Autodesk Inventor part; units mm, degrees
ref_plane "YZ Plane" through (0, 0, 0) normal (1, 0, 0) x (0, 1, 0)
ref_plane "XZ Plane" through (0, 0, 0) normal (0, 1, 0) x (-1, 0, 0)
ref_plane "XY Plane" through (0, 0, 0) normal (0, 0, 1) x (1, 0, 0)
sketch "Boceto1" plane through (0, 0, 0) normal (0, 0, 1) x (1, 0, 0)
  line L0 (0, 0) -> (127.5, 0)
  line L1 (127.5, 0) -> (127.5, 177)
  line L2 (127.5, 177) -> (0, 177)
  line L3 (0, 177) -> (0, 0)
  dimension "d32" = 127.5
  dimension "d33" = 177
extrude "Extrusión1" add sketch "Boceto1" along normal blind 2.5
sketch "Boceto2" plane through (0, 0, 2.5) normal (0, 0, 1) x (1, 0, 0)
  line L0 (127.5, 0) -> (127.5, 27.5)
  line L1 (127.5, 0) -> (127.5, 177)
  line L2 (127.5, 0) -> (155, 0) construction
  line L3 (127.5, 27.5) -> (113.75, 27.5)
  line L4 (0, 0) -> (127.5, 0)
  line L5 (113.75, 27.5) -> (13.75, 27.5)
  line L6 (13.75, 27.5) -> (13.75, 149.5)
  line L7 (13.75, 149.5) -> (113.75, 149.5)
  line L8 (113.75, 149.5) -> (113.75, 27.5)
  dimension "d36" = 27.5
  dimension "d37" = 90
  dimension "d38" = 13.75
  dimension "d39" = 90
  dimension "d40" = 100
  dimension "d41" = 122
extrude "Extrusión2" cut sketch "Boceto2" against normal blind 2.5
sketch "Boceto3" plane through (0, 0, 2.5) normal (0, 0, 1) x (1, 0, 0)
  line L0 (13.75, 149.5) -> (7.75, 149.5)
  line L1 (7.75, 149.5) -> (7.75, 155.5)
  line L2 (113.75, 27.5) -> (113.75, 21.5)
  line L3 (113.75, 27.5) -> (119.75, 27.5) construction
  line L4 (113.75, 21.5) -> (119.75, 21.5)
  line L5 (7.75, 155.5) -> (119.75, 155.5)
  line L6 (119.75, 155.5) -> (119.75, 21.5)
  line L7 (119.75, 21.5) -> (7.75, 21.5)
  line L8 (7.75, 21.5) -> (7.75, 155.5)
  line L9 (0, 177) -> (127.5, 177)
  line L10 (127.5, 177) -> (127.5, 0)
  line L11 (127.5, 0) -> (0, 0)
  line L12 (0, 0) -> (0, 177)
  dimension "d44" = 6
  dimension "d45" = 6
  dimension "d46" = 90
  dimension "d47" = 6
  dimension "d48" = 90
  dimension "d49" = 6
  dimension "d50" = 90
extrude "Extrusión3" add sketch "Boceto3" along normal blind 6
sketch "Boceto6" plane through (0, 0, 8.5) normal (0, 0, 1) x (1, 0, 0)
  line L0 (0, 0) -> (0, 88.5)
  line L1 (0, 177) -> (0, 0)
  line L2 (0, 0) -> (88.5, 0) construction
  line L3 (0, 88.5) -> (127.5, 88.5)
  dimension "d73" = 88.5
  dimension "d74" = 90
  dimension "d75" = 127.5
  dimension "d76" = 90
ref_plane "Plano de trabajo1" through (0, 88.5, 8.5) normal (0, -1, 0) x (1, 0, 0)
sketch "Boceto7" plane through (0, 0, 8.5) normal (0, 0, 1) x (1, 0, 0)
  line L0 (0, 0) -> (63.75, 0)
  line L1 (0, 0) -> (127.5, 0)
  line L2 (63.75, 0) -> (63.75, 177)
  line L3 (127.5, 177) -> (0, 177)
  line L4 (63.75, 0) -> (240.75, 0) construction
  dimension "d78" = 177
  dimension "d79" = 90
ref_plane "Plano de trabajo2" through (63.75, 0, 8.5) normal (1, 0, 0) x (0, 1, 0)
sketch "Boceto8" plane through (0, 0, 2.5) normal (0, 0, 1) x (1, 0, 0)
  line L0 (13.75, 27.5) -> (7.75, 27.5)
  line L1 (7.75, 27.5) -> (7.75, 21.5)
  line L2 (7.75, 21.5) -> (13.75, 21.5)
  line L3 (13.75, 21.5) -> (13.75, 27.5)
  line L4 (13.75, 21.5) -> (7.75, 27.5)
  line L5 (13.75, 27.5) -> (7.75, 21.5)
  circle A0 centre (10.75, 24.5) radius 1.6
  point P0 (0, 0)
  dimension "d81" = 6
  dimension "d82" = 6
  dimension "d83" = 3.2
extrude "Extrusión4" cut sketch "Boceto8" against normal blind 4 contours A0 L4 L5 | L5 L4 A0 | L4 L5 A0 | A0 L5 L4
mirror "Simetría1" about plane through (63.75, 0, 8.5) normal (1, 0, 0) of "Extrusión4"
mirror "Simetría2" about plane through (0, 88.5, 8.5) normal (0, -1, 0) of "Extrusión4", "Simetría1"
sketch "Boceto9" plane through (0, 0, 8.5) normal (0, 0, 1) x (1, 0, 0)
  line L0 (0, 177) -> (11.5, 177)
  line L1 (11.5, 177) -> (11.5, 165.5)
  line L2 (11.5, 165.5) -> (0, 165.5)
  line L3 (0, 165.5) -> (0, 177)
  line L4 (0, 177) -> (11.5, 165.5)
  line L5 (0, 165.5) -> (11.5, 177)
  circle A0 centre (5.75, 171.25) radius 2.1
  point P0 (0, 0)
  dimension "d86" = 11.5
  dimension "d87" = 11.5
  dimension "d88" = 4.2
extrude "Extrusión5" cut sketch "Boceto9" against normal blind 10 contours A0 L5 L4 | L4 L5 A0 | A0 L4 L5 | L5 L4 A0
mirror "Simetría3" about plane through (63.75, 0, 8.5) normal (1, 0, 0) of "Extrusión5"
mirror "Simetría4" about plane through (0, 88.5, 8.5) normal (0, -1, 0) of "Extrusión5", "Simetría3"
properties part number "transillum_diffusor_partA_v3"
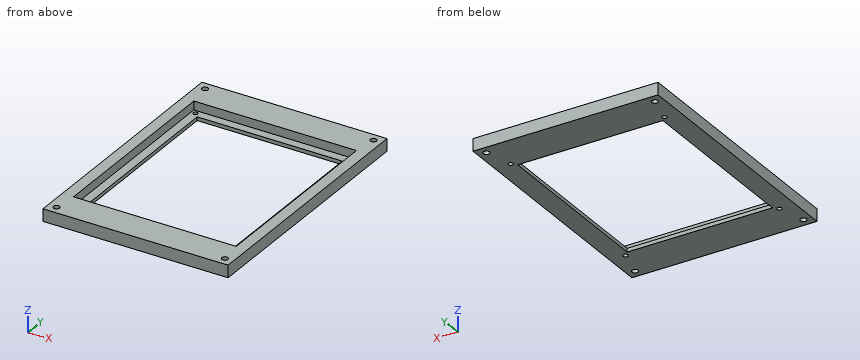
Can you work these out from the model? Positions are in its coordinate system, mm. Round coordinates to 2 decimals unless told otherwise and drop trailing zeros. Write each loop counter-clockwise with the first axis right and the second up, starting at its lowest first coordinate (ties: lowest second). Pieces come first, ordered by that corner, then holes. Notation, with made-up numbers: (35.5, -7) -> (71.5, -7) arc R24 ccw to (71.5, 23) -> close; hole circle Ø9 at (31, 21). An arc over 180 degrees is marked (long way). One line per question, with ' | ' between items. Start each with the question number.
1) Suppose I cut it at A-A on x = 107. Write out the boundary of the cut face in (y, z), then the cut area to 4 significant figures.
2) I need wall thicknesses on line 1 (Y direction, x = 5.75, z = 4); line 2 (X direction, y = 171.25, z = 5.5); line 3 (Y direction, x = 10.75, z = 1.75). Which ranges of each line are inside material? Lowest first, please. Write a range as [from, to].
3) I'm going to push flat-ended pins straight in: P1, Ø4, axis at x = 10.75, y = 152.5, coming from the -Z side; P2, Ø1, axis at x = 16, y = 153.5, coming from the +Z side. Where does each tip first touch, or does it pass through?
4) Suppose I cut it at C-C on y = 89. Write out the boundary of the cut face in (x, z), then the cut area to 3 significant figures.
5) Suppose I cut it at B-B on y = 5.75. Write out the boundary of the cut face in (x, z), then the cut area to 3 significant figures.
Return value:
1) outline: (0, 0) -> (27.5, 0) -> (27.5, 2.5) -> (21.5, 2.5) -> (21.5, 8.5) -> (0, 8.5) -> close; (149.5, 0) -> (177, 0) -> (177, 8.5) -> (155.5, 8.5) -> (155.5, 2.5) -> (149.5, 2.5) -> close | area: 395.5 mm2
2) line 1: y = [0, 3.65], [7.85, 169.15], [173.35, 177] | line 2: x = [0, 3.65], [7.85, 119.65], [123.85, 127.5] | line 3: y = [0, 22.9], [26.1, 150.9], [154.1, 177]
3) P1: stops at z = 0 | P2: stops at z = 2.5
4) outline: (0, 0) -> (13.75, 0) -> (13.75, 2.5) -> (7.75, 2.5) -> (7.75, 8.5) -> (0, 8.5) -> close; (113.75, 0) -> (127.5, 0) -> (127.5, 8.5) -> (119.75, 8.5) -> (119.75, 2.5) -> (113.75, 2.5) -> close | area: 162 mm2
5) outline: (0, 0) -> (3.65, 0) -> (3.65, 8.5) -> (0, 8.5) -> close; (7.85, 0) -> (119.65, 0) -> (119.65, 8.5) -> (7.85, 8.5) -> close; (123.85, 0) -> (127.5, 0) -> (127.5, 8.5) -> (123.85, 8.5) -> close | area: 1,010 mm2
